The model under review builds one solid part; all positions refer to its coordinate system, in mm. A direction names the side the tool comes from. Round coordinates to 2 decimals unless told otherwise and drop trailing zeros. Write each loop counter-clockwise with the first axis right and the second up, starting at its lowest first coordinate (ties: lowest second). Pieces come first, ordered by that corner, then holes. Notation, with made-up numbers: (-38.5, 76) -> (14.5, 76) arc R9 cw to (14.5, 93) -> close; hole circle Ø7 at (-19.75, -7). An arc over 180 degrees is marked (long way). Answer in a Markdown table with one row per item. Add a question column.
```python
from build123d import *

# Parameters (mm, degrees)
SKETCH1_W                  = 25.4
SKETCH1_H                  = 25.4
SKETCH1_W_2                = 22.225
SKETCH1_H_2                = 22.225
BOSS_EXTRUDE1_DEPTH        = 685.8
F_7_0_201_DIAMETER_HOLE1_D = 5.1054
F_7_0_201_DIAMETER_HOLE2_D = 5.1054


with BuildPart() as part:
    # Sketch1 → Boss-Extrude1 (new body)
    with BuildSketch(Plane(origin=(0, 0, 0), x_dir=(1, 0, 0), z_dir=(0, 1, 0))):
        Rectangle(SKETCH1_W, SKETCH1_H)
        Rectangle(SKETCH1_W_2, SKETCH1_H_2, mode=Mode.SUBTRACT)
    extrude(amount=BOSS_EXTRUDE1_DEPTH)

    # #7 (0.201) Diameter Hole1 (through all)
    with Locations(Plane.XY.offset(12.7)):
        with Locations((0, 292.1), (0, 317.5), (0, 342.9), (0, 368.3), (0, 393.7)):
            Hole(F_7_0_201_DIAMETER_HOLE1_D / 2)

    # #7 (0.201) Diameter Hole2 (through all)
    with Locations(Plane(origin=(12.7, 0, 0), x_dir=(0, 0, -1), z_dir=(1, 0, 0))):
        with Locations((0, 12.7), (0, 38.1), (0, 622.3), (0, 647.7), (0, 673.1), (0, 596.9), (0, 546.1), (0, 520.7), (0, 469.9), (0, 419.1)):
            Hole(F_7_0_201_DIAMETER_HOLE2_D / 2)


solid = part.part
```
1. For L1, parallel to Y at x = 0, z = 12.25; L2, parallel to Z at x = -2.75, y = 370; L3, parallel to X at y = 342.9, z = 12.25, list the stretches that pass through material, from the lowest coordinate up.
2. Tool access review of faces 4 (the flat face through (-11.112, 338, 0)), 5 (the flat face through (-11.3, 685.8, -0.1)): name each direction out of +Z, -Z, +X, -X, +Y, -Y from which nothing blocks a thin tool from reaching the whole face with its end or side.
3. Add section B-B on y = 529.5. Write out the cut boundary in (x, z).
4. Mouldability with a two-part tool opening along X and no side actions: class faces 1 (the flat face through (12.7, 338, 0)), 2 (the flat face through (-11.3, 0, -0.1)), 3 (the flat face through (11.112, 338, 0)) as pulls with the +X half, pulls with the -X half, needs draft (parallel to the pull), parting line crosses it, or undercut.
5. Insertion check: pin 1 Ø6.5 at (x, y) = (0, 368.3) entering from -Z; pin 2 Ø3 at (y, z) = (546.1, 0) entering from +X. Each pin has a flat end and moves straight along its axis. Give the tip position at first contact, or say it passes through.
6. Add section A-A on z = 7.25. Write out the cut boundary in (x, y).
Filled in:
| question | item | result |
|---|---|---|
| 1 | L1 | 0 to 289.55, 294.65 to 314.95, 320.05 to 340.35, 345.45 to 365.75, 370.85 to 391.15, 396.25 to 685.8 |
| 1 | L2 | -12.7 to -11.11, 11.11 to 12.7 |
| 1 | L3 | -12.7 to -2.55, 2.55 to 12.7 |
| 2 | face 4 | +Y, -Y |
| 2 | face 5 | +Z, -Z, +X, -X, +Y |
| 3 | outline | (-12.7, -12.7) -> (12.7, -12.7) -> (12.7, 12.7) -> (-12.7, 12.7) -> close; hole (-11.11, -11.11) -> (11.11, -11.11) -> (11.11, 11.11) -> (-11.11, 11.11) -> close |
| 4 | face 1 | pulls with the +X half |
| 4 | face 2 | needs draft |
| 4 | face 3 | undercut |
| 5 | pin 1 | z = -12.7 |
| 5 | pin 2 | through |
| 6 | outline | (-12.7, 0) -> (-11.11, 0) -> (-11.11, 685.8) -> (-12.7, 685.8) -> close; (11.11, 0) -> (12.7, 0) -> (12.7, 685.8) -> (11.11, 685.8) -> close |
